from build123d import *

# Parameters (mm, degrees)
F0_W           = 120
F0_H           = 80
F1_DEPTH       = 25
F2_T           = -2.5
F4_D           = 5
F4_DEPTH       = 12
F4_CSINK_D     = 10
F4_CSINK_ANGLE = 90
F5_D           = 5
F5_DEPTH       = 12
F5_CSINK_D     = 10
F5_CSINK_ANGLE = 90


with BuildPart() as f1:
    # F0 (on Top) → F1 (new body)
    with BuildSketch(Plane.XY):
        with Locations((5.008996, -1.665502)):
            Rectangle(F0_W, F0_H)
    extrude(amount=F1_DEPTH)

    # F2
    f2_openings = [f1.faces().sort_by_distance(p)[0] for p in [
        (5.008996, -1.665502, 25),
    ]]
    offset(amount=F2_T, openings=f2_openings)

    # F4
    with Locations(Plane.XZ.offset(41.665502)):
        with Locations((-34.991004, 12.5)):
            CounterSinkHole(F4_D / 2, F4_CSINK_D / 2, depth=F4_DEPTH, counter_sink_angle=F4_CSINK_ANGLE)

    # F5
    with Locations(Plane.XZ.offset(41.665502)):
        with Locations((45.008996, 12.5)):
            CounterSinkHole(F5_D / 2, F5_CSINK_D / 2, depth=F5_DEPTH, counter_sink_angle=F5_CSINK_ANGLE)


solid = f1.part
Design review of the part built by this model. Coordinates are the model's own, in mm. A direction names the side the tool comes from. Coordinates: 2 decimals unless noted, no trailing zeros. Write each loop counter-clockwise with the first axis right and the second up, starting at its lowest first coordinate (ties: lowest second). Pieces come first, ordered by that corner, then holes. Notation, with made-up numbers: (89, 30) - (101, 30) arc R21 cw to (101, 57) - close; hole circle Ø11 at (-27.5, 52). An arc over 180 degrees is marked (long way). One line per item, written item: value.
1) To check wall thickness, follow probe 1 along Y at (x, z) = (-25, 13); probe 2 along X at (y, z) = (24.5, 15.75); probe 3 along Z at (x, y) = (-45.5, 30). State the ranges of each line that lie inside material, in increasing order.
Answer sheet:
probe 1: y = -41.67 to -39.17, 35.83 to 38.33
probe 2: x = -54.99 to -52.49, 62.51 to 65.01
probe 3: z = 0 to 2.5
2) Mouldability with a two-part tool opening along X and no side actions: class faces 1 (the face through (-54.991, -2, 12)), 2 (the face through (4, -1, 0)), 3 (the face through (4, -39.166, 14)) as +X half, -X half, draft (parallel to the pull), parting line (faces both ways), or undercut.
Answer sheet:
face 1: -X half
face 2: draft
face 3: undercut
3) For faces 4 (the face through (65.009, -2, 12)), 5 (the face through (62.509, -2, 14)), list the 3-axis set-ups (+Z, -Z, +X, -X, +Y, -Y) from which the entire face can be reached by the end or side of a thin tool; tool diameter is ignored.
Answer sheet:
face 4: +Z, -Z, +X, +Y, -Y
face 5: +Z
4) Add section C-C (x = 14.5). State the section outline as (y, z) points.
Answer sheet:
outline: (-41.67, 0) - (38.33, 0) - (38.33, 25) - (35.83, 25) - (35.83, 2.5) - (-39.17, 2.5) - (-39.17, 25) - (-41.67, 25) - close
5) Add section B-B (y = 22.5). State the section outline as (x, z) points.
Answer sheet:
outline: (-54.99, 0) - (65.01, 0) - (65.01, 25) - (62.51, 25) - (62.51, 2.5) - (-52.49, 2.5) - (-52.49, 25) - (-54.99, 25) - close
6) Insertion check: pin 1 (22.5 mm diameter, centred on x = -7.5, y = 0.5, fed in from +Z). The pin has a flat end and moves straight along its axis. Give the tip position at first contact, or say it passes through.
Answer sheet:
pin 1: stops at z = 2.5
7) Add section A-A (z = 12.5). State the section outline as (x, y) points, plus the area to 4 significant figures.
Answer sheet:
outline: (-54.99, -41.67) - (-39.99, -41.67) - (-37.49, -39.17) - (-52.49, -39.17) - (-52.49, 35.83) - (62.51, 35.83) - (62.51, -39.17) - (47.51, -39.17) - (50.01, -41.67) - (65.01, -41.67) - (65.01, 38.33) - (-54.99, 38.33) - close; (-32.49, -39.17) - (-29.99, -41.67) - (40.01, -41.67) - (42.51, -39.17) - close
area: 937.5 mm2
8) Add section D-D (z = 19.75). State the section outline as (x, y) points.
Answer sheet:
outline: (-54.99, -41.67) - (65.01, -41.67) - (65.01, 38.33) - (-54.99, 38.33) - close; hole (-52.49, -39.17) - (62.51, -39.17) - (62.51, 35.83) - (-52.49, 35.83) - close
